Geometry check sheet. Reference: the model listing, model coordinates, mm. Coordinates: 2 decimals unless noted, no trailing zeros. Loops run counter-clockwise (first coordinate to the right, second up) from the corner with the lowest first, then second, coordinate; pieces in that order, holes last. Notation, with made-up numbers: (-38, -38) -> (19, -38) arc R15 ccw to (19, -21) -> close; hole circle Ø10 at (11.5, 78). An arc over 180 degrees is marked (long way). Answer as a JSON object with one key per item and string values.
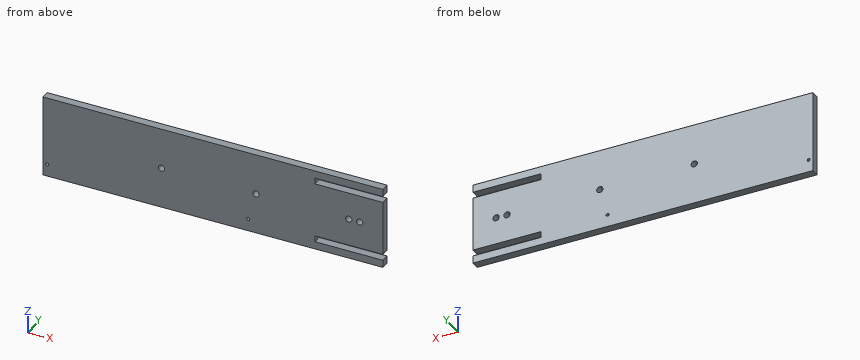
from build123d import *

# Parameters (mm, degrees)
SKETCH1_W           = 250
SKETCH1_H           = 60
SKETCH1_R           = 2.3
BOSS_EXTRUDE1_DEPTH = 6
SKETCH2_W           = 50
SKETCH2_H           = 4.5
CUT_EXTRUDE1_DEPTH  = 6
SKETCH3_R           = 1.1
CUT_EXTRUDE2_DEPTH  = 10


with BuildPart() as part:
    # Sketch1 → Boss-Extrude1 (new body)
    with BuildSketch(Plane(origin=(0, 0, 0), x_dir=(1, 0, 0), z_dir=(0, 1, 0))):
        Rectangle(SKETCH1_W, SKETCH1_H)
        with Locations((108, 0)):
            Circle(SKETCH1_R, mode=Mode.SUBTRACT)
        with Locations((100, 0)):
            Circle(SKETCH1_R, mode=Mode.SUBTRACT)
        with Locations((31.7, 0)):
            Circle(SKETCH1_R, mode=Mode.SUBTRACT)
        with Locations((-37.8, 0)):
            Circle(SKETCH1_R, mode=Mode.SUBTRACT)
    extrude(amount=BOSS_EXTRUDE1_DEPTH)

    # Sketch2 → Cut-Extrude1 (cut)
    with BuildSketch(Plane(origin=(0, 6, 0), x_dir=(1, 0, 0), z_dir=(0, 1, 0))):
        with Locations((100, -22.25)):
            Rectangle(SKETCH2_W, SKETCH2_H)
        with Locations((100, 22.25)):
            Rectangle(SKETCH2_W, SKETCH2_H)
    extrude(amount=-CUT_EXTRUDE1_DEPTH, mode=Mode.SUBTRACT)

    # Sketch3 → Cut-Extrude2 (cut)
    with BuildSketch(Plane.XZ):
        with Locations((-122, -21)):
            Circle(SKETCH3_R)
        with Locations((26, -21)):
            Circle(SKETCH3_R)
    extrude(amount=-CUT_EXTRUDE2_DEPTH, mode=Mode.SUBTRACT)


solid = part.part
1. Thickness scan on probe 1 along Z at (x, y) = (90.5, 1.35); probe 2 along Z at (x, y) = (108, 2.3); probe 3 along X at (y, z) = (3.4, 0). Record the ranges inside material, lowest first. Write a range as from..to.
Evaluation:
{"probe 1": "z = -30..-24.5, -20..20, 24.5..30", "probe 2": "z = -30..-24.5, -20..-2.3, 2.3..20, 24.5..30", "probe 3": "x = -125..-40.1, -35.5..29.4, 34..97.7, 102.3..105.7, 110.3..125"}
2. Section check C-C, the plane x = -37.8. Record the boundary of the cut face in (y, z).
Evaluation:
{"outline": "(0, -30) -> (6, -30) -> (6, -2.3) -> (0, -2.3) -> close; (0, 2.3) -> (6, 2.3) -> (6, 30) -> (0, 30) -> close"}
3. Section check B-B, the plane y = 3.9. Record the boundary of the cut face in (x, z).
Evaluation:
{"outline": "(-125, -30) -> (125, -30) -> (125, -24.5) -> (75, -24.5) -> (75, -20) -> (125, -20) -> (125, 20) -> (75, 20) -> (75, 24.5) -> (125, 24.5) -> (125, 30) -> (-125, 30) -> close; hole circle Ø2.2 at (-122, -21); hole circle Ø4.6 at (-37.8, 0); hole circle Ø2.2 at (26, -21); hole circle Ø4.6 at (31.7, 0); hole circle Ø4.6 at (100, 0); hole circle Ø4.6 at (108, 0)"}
4. Depth check by flat-ended pin: P1, Ø7.5, axis at x = -37.8, z = 0, coming from the +Y side; P2, Ø1.3, axis at y = 4.5, z = -22, coming from the +X side. Enter the tip coordinate at first touch or a pass-through.
Evaluation:
{"P1": "stops at y = 6", "P2": "stops at x = 75"}
5. Section check A-A, the plane x = 84.5. Record the boundary of the cut face in (y, z), then the cut area to 3 significant figures.
Evaluation:
{"outline": "(0, -30) -> (6, -30) -> (6, -24.5) -> (0, -24.5) -> close; (0, -20) -> (6, -20) -> (6, 20) -> (0, 20) -> close; (0, 24.5) -> (6, 24.5) -> (6, 30) -> (0, 30) -> close", "area": "306 mm^2"}
